from build123d import *

# Parameters (mm, degrees)
BOSS_EXTRUDE1_DEPTH = 12
SKETCH2_R           = 1.65
CUT_EXTRUDE1_DEPTH  = 12
SKETCH3_W           = 7
SKETCH3_H           = 7
SKETCH3_R           = 1.65
BOSS_EXTRUDE2_DEPTH = 3


with BuildPart() as part:
    # Sketch1 → Boss-Extrude1 (new body)
    with BuildSketch(Plane(origin=(0, 0, 0), x_dir=(1, 0, 0), z_dir=(0, 1, 0))):
        Polygon((7.5, -7.5), (7.5, 7.5), (-7.5, 7.5), (-7.5, -7.5), (-17.5, -7.5), (-17.5, -4.5), (-10.5, -4.5), (-10.5, 10.5), (10.5, 10.5), (10.5, -4.5), (17.5, -4.5), (17.5, -7.5), align=None)
    extrude(amount=BOSS_EXTRUDE1_DEPTH)

    # Sketch2 → Cut-Extrude1 (cut)
    with BuildSketch(Plane.XY.offset(7.5)):
        with Locations((-14, 6)):
            Circle(SKETCH2_R)
        with Locations((14, 6)):
            Circle(SKETCH2_R)
    extrude(amount=-CUT_EXTRUDE1_DEPTH, mode=Mode.SUBTRACT)

    # Sketch3 → Boss-Extrude2 (add)
    with BuildSketch(Plane(origin=(0, 12, 0), x_dir=(1, 0, 0), z_dir=(0, 1, 0))):
        with Locations((-14, 3.5)):
            Rectangle(SKETCH3_W, SKETCH3_H)
        with Locations((-14, 3.5)):
            Circle(SKETCH3_R, mode=Mode.SUBTRACT)
        with Locations((14, 3.5)):
            Rectangle(SKETCH3_W, SKETCH3_H)
        with Locations((14, 3.5)):
            Circle(SKETCH3_R, mode=Mode.SUBTRACT)
    extrude(amount=-BOSS_EXTRUDE2_DEPTH)


solid = part.part
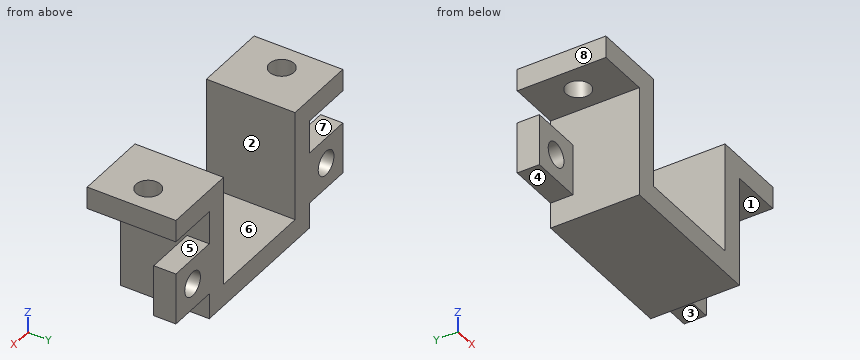
CAD build for the part. Positions are in the model's coordinates, mm. Face numbers are marked on the shaded views. A direction names the side the tool comes from. Coordinates: 2 decimals unless noted, no trailing zeros. Write each loop counter-clockwise with the first axis right and the second up, starting at its lowest first coordinate (ties: lowest second). Pieces come first, ordered by that corner, then holes. Notation, with made-up numbers: M 1.5,62 L 22.5,62 A28 ccw 22.5,96 Z; hole C -22,-20.5 d2. An arc over 180 degrees is marked long. Answer as a JSON object with one key per item and string values. Group by question number.
1) Wall check: line 1 (X direction, y = 10.4, z = -3.5); line 2 (Z direction, x = -14, y = 10.5); line 3 (Y direction, x = 14, z = 5.7). Give the ranges that are in metal, low to high. Write a range as from..to.
2) Saw through at D-D (z = -3.5). Write the cut outline in (x, y).
3) Saw through at A-A (z = -1.25). Write the cut outline in (x, y).
4) Saw through at B-B (x = 14). Write the cut outline in (y, z).
5) Pin check, flat tips, straight feed: pin 1 Ø2 at (x, z) = (12.5, -5) entering from -Y; pin 2 Ø6 at (x, y) = (3.5, 8) entering from +Z; pin 3 Ø2 at (x, y) = (12.5, 5.5) entering from -Z. Stop position of each tip, or through.
6) Tool access for the marked faces 1, 2, 3 and 4: list every direction of +Z, -Z, +X, -X, +Y, -Y with a clear straight run to the whole face (end or side of a thin tool).
7) Mould opens along Z. For the marked faces 5, 6, 7 and 8 say: +Z half, -Z half, draft (parallel to the pull), parting line (faces both ways), or undercut.
8) Saw through at C-C (y = 11). Write the cut outline in (x, z), plus the area to 3 significant figures.
Values follow:
{
 "1": {"line 1": "x = -17.5..-15.65, -12.35..-7.5, 7.5..12.35, 15.65..17.5", "line 2": "z = -7..-5.15, -1.85..0, 4.5..7.5", "line 3": "y = 0..4.35, 7.65..12"},
 "2": {"outline": "M -17.5,9 L -15.65,9 L -15.65,12 L -17.5,12 Z; M -12.35,9 L -10.5,9 L -10.5,0 L -7.5,0 L -7.5,12 L -12.35,12 Z; M 7.5,0 L 10.5,0 L 10.5,9 L 12.35,9 L 12.35,12 L 7.5,12 Z; M 15.65,9 L 17.5,9 L 17.5,12 L 15.65,12 Z"},
 "3": {"outline": "M -17.5,9 L -10.5,9 L -10.5,0 L -7.5,0 L -7.5,12 L -17.5,12 Z; M 7.5,0 L 10.5,0 L 10.5,9 L 17.5,9 L 17.5,12 L 7.5,12 Z"},
 "4": {"outline": "M 0,4.5 L 4.35,4.5 L 4.35,7.5 L 0,7.5 Z; M 7.65,4.5 L 12,4.5 L 12,7.5 L 7.65,7.5 Z; M 9,-7 L 12,-7 L 12,-5.15 L 9,-5.15 Z; M 9,-1.85 L 12,-1.85 L 12,0 L 9,0 Z"},
 "5": {"pin 1": "stops at y = 9", "pin 2": "stops at z = -7.5", "pin 3": "stops at z = 4.5"},
 "6": {"face 1": "+X, +Y, -Y", "face 2": "+Z, +Y, -Y", "face 3": "-Z, +X, +Y, -Y", "face 4": "-Z, -X, +Y, -Y"},
 "7": {"face 5": "undercut", "face 6": "+Z half", "face 7": "undercut", "face 8": "draft"},
 "8": {"outline": "M -17.5,-7 L -10.5,-7 L -10.5,-10.5 L 10.5,-10.5 L 10.5,-7 L 17.5,-7 L 17.5,0 L 10.5,0 L 10.5,4.5 L 17.5,4.5 L 17.5,7.5 L 7.5,7.5 L 7.5,-7.5 L -7.5,-7.5 L -7.5,7.5 L -17.5,7.5 L -17.5,4.5 L -10.5,4.5 L -10.5,0 L -17.5,0 Z; hole C -14,-3.5 d3.3; hole C 14,-3.5 d3.3", "area": "276 mm2"}
}
